Design review of the part built by this model. Coordinates are the model's own, in mm. A direction names the side the tool comes from. Round coordinates to 2 decimals unless told otherwise and drop trailing zeros. Write each loop counter-clockwise with the first axis right and the second up, starting at its lowest first coordinate (ties: lowest second). Pieces come first, ordered by that corner, then holes. Notation, with made-up numbers: (-8, 2) -> (22, 2) arc R28 ccw to (22, 41) -> close; hole circle Ø8 at (49, 64.25). An arc over 180 degrees is marked (long way). Write item = value, one per line. Start each with the question number.
Item 1: Mouldability with a two-part tool opening along Y and no side actions: class faces 1 (the flat face through (200, 10, -15)), 2 (the cylindrical face through (4.93, -53.692, 11.923)), 3 (the cylindrical face through (98.6, -10.648, -13.887)) as released by +Y, released by -Y, zero draft, split by the parting line, or undercut.
Item 2: Machinability: for faces 4 (the flat face through (193, -32, -10)), 5 (the flat face through (193, -43, 0)), 6 (the flat face through (193, 32, 10)), 7 (the flat face through (193, -32, 10)), which of the approach directions +Z, -Z, +X, -X, +Y, -Y give a long, thin tool a straight path to every point of the face, cutting with its end or side? Answer none if there is none.
Item 3: Add section C-C, the plane x = 142.5. State the section outline as (y, z) points.
Item 4: To check wall thickness, follow L1, parallel to Y at x = 68, z = 0; L2, parallel to X at y = -28, z = -32; L3, parallel to Z at x = 13, y = 12. State the ranges of each line that lie inside material, in increasing order.
Item 5: Add section B-B, the plane y = 0. State the section outline as (x, z) points.
Item 6: Add section A-A, the plane z = 0. State the section outline as (x, y) points, then the cut area to 4 significant figures.
Item 7: Add section D-D, the plane y = -30. State the section outline as (x, z) points, then the cut area to 3 significant figures.
Item 8: For pin 1 Ø8 at (x, z) = (61, -21) entering from +Y; pin 2 Ø0.6 at (x, z) = (191.5, 9.5) entering from -Y; pin 3 Ø4.5 at (x, y) = (189, -36.5) entering from -Z; pin 4 Ø16 at (y, z) = (-29.5, -3) entering from -X, all flat-tipped, find the tip position at first contact; note any pin that passes through.
from build123d import *

# Parameters (mm, degrees)
SKETCH2_R               = 55
BOSS_EXTRUDE1_DEPTH     = 10
SKETCH3_R               = 22.5
BOSS_EXTRUDE2_DEPTH     = 190
SKETCH4_R               = 17.5
CUT_EXTRUDE1_DEPTH      = 1
CUT_EXTRUDE1_DEPTH_BACK = 201
SKETCH9_W               = 20
SKETCH9_H               = 22
BOSS_EXTRUDE3_DEPTH     = 15
SKETCH10_W              = 20
SKETCH10_H              = 23
BOSS_EXTRUDE4_DEPTH     = 15


with BuildPart() as part:
    # Sketch2 → Boss-Extrude1 (new body)
    with BuildSketch(Plane(origin=(0, 0, 0), x_dir=(0, 0, -1), z_dir=(1, 0, 0))):
        Circle(SKETCH2_R)
    extrude(amount=BOSS_EXTRUDE1_DEPTH)

    # Sketch3 → Boss-Extrude2 (add)
    with BuildSketch(Plane(origin=(10, 0, 0), x_dir=(0, 0, -1), z_dir=(1, 0, 0))):
        Circle(SKETCH3_R)
    extrude(amount=BOSS_EXTRUDE2_DEPTH)

    # Sketch4 → Cut-Extrude1 (cut, two sides)
    with BuildSketch(Plane.ZY) as cut_extrude1_sk:
        Circle(SKETCH4_R)
    extrude(amount=CUT_EXTRUDE1_DEPTH, mode=Mode.SUBTRACT)
    extrude(cut_extrude1_sk.sketch, amount=-CUT_EXTRUDE1_DEPTH_BACK, mode=Mode.SUBTRACT)

    # Sketch9 → Boss-Extrude3 (add)
    with BuildSketch(Plane(origin=(200, 0, 0), x_dir=(0, 0, -1), z_dir=(1, 0, 0))):
        with Locations((0, 32)):
            Rectangle(SKETCH9_W, SKETCH9_H)
    extrude(amount=-BOSS_EXTRUDE3_DEPTH)

    # Sketch10 → Boss-Extrude4 (add)
    with BuildSketch(Plane(origin=(200, 0, 0), x_dir=(0, 0, -1), z_dir=(1, 0, 0))):
        with Locations((0, -31.5)):
            Rectangle(SKETCH10_W, SKETCH10_H)
    extrude(amount=-BOSS_EXTRUDE4_DEPTH)


solid = part.part
Result set:
q1.face_1 = zero draft
q1.face_2 = split by the parting line
q1.face_3 = undercut
q2.face_4 = -Z, +X, -Y
q2.face_5 = +Z, -Z, +X, -Y
q2.face_6 = +Z, +X, +Y
q2.face_7 = +Z, +X, -Y
q3.outline = circle Ø45 at (0, 0); hole circle Ø35 at (0, 0)
q4.L1 = -22.5 to -17.5, 17.5 to 22.5
q4.L2 = 0 to 10
q4.L3 = -19.03 to -12.74, 12.74 to 19.03
q5.outline = (0, -55) -> (10, -55) -> (10, -22.5) -> (200, -22.5) -> (200, -17.5) -> (0, -17.5) -> close; (0, 17.5) -> (200, 17.5) -> (200, 22.5) -> (10, 22.5) -> (10, 55) -> (0, 55) -> close
q6.outline = (0, -55) -> (10, -55) -> (10, -22.5) -> (185, -22.5) -> (185, -43) -> (200, -43) -> (200, -17.5) -> (0, -17.5) -> close; (0, 17.5) -> (200, 17.5) -> (200, 43) -> (185, 43) -> (185, 22.5) -> (10, 22.5) -> (10, 55) -> (0, 55) -> close
q6.area = 3,265 mm²
q7.outline = (0, -46.1) -> (10, -46.1) -> (10, 46.1) -> (0, 46.1) -> close; (185, -10) -> (200, -10) -> (200, 10) -> (185, 10) -> close
q7.area = 1,220 mm²
q8.pin_1 = 14.74
q8.pin_2 = -43
q8.pin_3 = -10
q8.pin_4 = 0
